Can you work these out from the model? Positions are in its coordinate system, mm. Face numbers are marked on the shaded views. A direction names the side the tool comes from. Round coordinates to 2 decimals unless told otherwise and drop trailing zeros. Loops run counter-clockwise (first coordinate to the right, second up) from the corner with the lowest first, then second, coordinate; pieces in that order, holes last. Notation, with made-up numbers: (-20, -37) -> (-3, -37) arc R12 cw to (-3, -28) -> close; hole circle Ø10 at (20, 22). An arc over 180 degrees is marked (long way). Write item = value, one per line.
Autodesk Inventor part; units mm, degrees
ref_plane "YZ Plane" through (0, 0, 0) normal (1, 0, 0) x (0, 1, 0)
ref_plane "XZ Plane" through (0, 0, 0) normal (0, 1, 0) x (-1, 0, 0)
ref_plane "XY Plane" through (0, 0, 0) normal (0, 0, 1) x (1, 0, 0)
sketch "Esquisse1" plane through (0, 0, 0) normal (0, 0, 1) x (1, 0, 0)
  line L0 (2, 0) -> (68, 0)
  line L1 (70, 2) -> (70, 28)
  line L2 (68, 30) -> (2, 30)
  line L3 (0, 28) -> (0, 2)
  arc A0 (2, 30) -> (0, 28) centre (2, 28) ccw
  arc A1 (70, 28) -> (68, 30) centre (68, 28) ccw
  arc A2 (68, 0) -> (70, 2) centre (68, 2) ccw
  arc A3 (0, 2) -> (2, 0) centre (2, 2) ccw
  point P0 (0, 0)
  point P1 (70, 30)
  point P2 (70, 0)
  point P3 (0, 30)
  dimension "d0" = 70
  dimension "d1" = 30
  dimension "d14" = 2
extrude "Extrusion1" add sketch "Esquisse1" along normal blind 5
sketch "Esquisse2" plane through (0, 0, 0) normal (-1, 0, 0) x (0, 0, 1)
  line L0 (5, 2) -> (5, 28)
  line L1 (5, 15) -> (5, 19)
  line L2 (5, 15) -> (5, 11)
  line L3 (5, 19) -> (11, 19)
  line L4 (13, 17) -> (13, 13)
  line L5 (11, 11) -> (5, 11)
  arc A0 (13, 17) -> (11, 19) centre (11, 17) ccw
  arc A1 (11, 11) -> (13, 13) centre (11, 13) ccw
  line L6 (5, 19) -> (12.4142, 11.5858) construction
  line L7 (5, 11) -> (12.4142, 18.4142) construction
  circle A2 centre (9, 15) radius 2.75
  line L8 (0, 2) -> (0, 28)
  line L9 (5, 2) -> (5, 28)
  line L10 (0, 2) -> (5, 2)
  line L11 (5, 28) -> (5, 2)
  line L12 (0, 28) -> (5, 28)
  line L13 (0, 2) -> (0, 28)
  line L14 (0, 2) -> (5, 2)
  line L15 (5, 28) -> (5, 2)
  line L16 (0, 28) -> (5, 28)
  line L17 (0, 2) -> (0, 28)
  line L18 (0, 28) -> (5, 28)
  line L19 (0, 2) -> (5, 2)
  point P0 (5, 0)
  point P1 (5, 30)
  point P2 (13, 19)
  dimension "d4" = 4
  dimension "d5" = 4
  dimension "d6" = 8
  dimension "d7" = 2
  dimension "d8" = 5.5
extrude "Extrusion2" add sketch "Esquisse2" against normal blind 5 contours L0 L3 A0 L4 A1 L5
sketch "Esquisse3" plane through (70, 0, 0) normal (1, 0, 0) x (0, 0, -1)
  line L0 (-11, 19) -> (-5, 19)
  line L1 (-5, 19) -> (-11, 19)
  line L2 (-11, 19) -> (-11, 19)
  line L3 (-13, 13) -> (-13, 17)
  line L4 (-13, 17) -> (-13, 13)
  line L5 (-11, 11) -> (-5, 11)
  line L6 (-5, 2) -> (-5, 28)
  line L7 (-5, 19) -> (-5, 11)
  arc A0 (-11, 19) -> (-13, 17) centre (-11, 17) ccw
  arc A1 (-13, 13) -> (-11, 11) centre (-11, 13) ccw
  circle A2 centre (-9, 15) radius 2.75
  circle A3 centre (-9, 15) radius 2.5
  point P0 (0, 0)
  point P1 (-13, 19)
  point P2 (-5, 0)
  point P3 (-5, 30)
  dimension "d11" = 2
extrude "Extrusion3" add sketch "Esquisse3" against normal blind 5 contours L0 L6 L5 A1 L3 A0
properties part number "Pied"
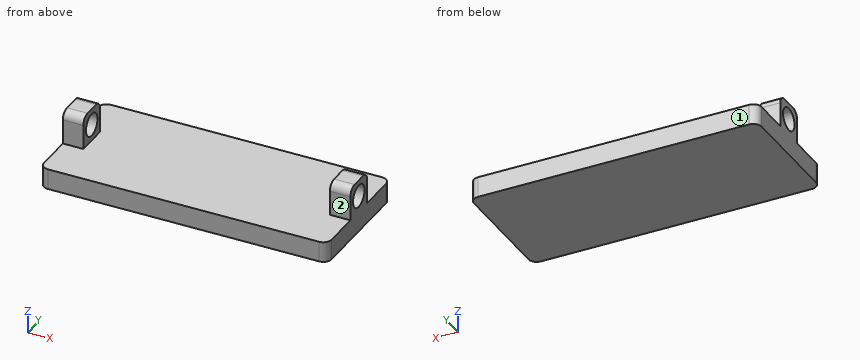
1. For the marked faces 1 and 2, which set-ups out of +Z, -Z, +X, -X, +Y, -Y let a thin tool reach every point of the face, with its end or its side?
Entries:
face_1 = +Z, -Z, +X, -X, +Y
face_2 = +Z, +X, -X, -Y
2. I need wall thicknesses on line 1 (X direction, y = 12.25, z = 11); line 2 (Y direction, x = 68.9, z = 9); line 3 (Z direction, x = 22, y = 15). Which ranges of each line are inside material? Lowest first, please. Write a range as [from, to].
Entries:
line_1 = [0, 5], [65, 70]
line_2 = [11, 12.25], [17.75, 19]
line_3 = [0, 5]
3. Suppose I cut it at A-A, the plane y = 15. List the corners of the cut face in (x, z) for me, and give its area (3 significant figures).
Entries:
outline = (0, 0) -> (70, 0) -> (70, 6.25) -> (65, 6.25) -> (65, 5) -> (5, 5) -> (5, 6.25) -> (0, 6.25) -> close; (0, 11.75) -> (5, 11.75) -> (5, 13) -> (0, 13) -> close; (65, 11.75) -> (70, 11.75) -> (70, 13) -> (65, 13) -> close
area = 375 mm²
4. Suppose I cut it at B-B, the plane z = 9. List the corners of the cut face in (x, y) for me.
Entries:
outline = (0, 11) -> (5, 11) -> (5, 12.25) -> (0, 12.25) -> close; (0, 17.75) -> (5, 17.75) -> (5, 19) -> (0, 19) -> close; (65, 11) -> (70, 11) -> (70, 12.25) -> (65, 12.25) -> close; (65, 17.75) -> (70, 17.75) -> (70, 19) -> (65, 19) -> close
5. Suppose I cut it at C-C, the plane x = 29.5. List the corners of the cut face in (y, z) for me.
Entries:
outline = (0, 0) -> (30, 0) -> (30, 5) -> (0, 5) -> close
6. Suppose I cut it at D-D, the plane y = 5.25. List the corners of the cut face in (x, z) for me, and give its area (3 significant figures).
Entries:
outline = (0, 0) -> (70, 0) -> (70, 5) -> (0, 5) -> close
area = 350 mm²
7. I'm going to push flat-ended pins straight in: pin 1 (4 mm diameter, centred on x = 3.5, z = 9.5, fed in from -Y); pin 2 (9 mm diameter, centred on x = 33.5, y = 17, fed in from +Z); pin 3 (2.5 mm diameter, centred on x = 67.5, z = 8.5, fed in from +Y); pin 4 (5.5 mm diameter, centred on x = 1.5, z = 7, fed in from +Y). Where does each tip first touch, or does it pass through?
Entries:
pin_1 = 11
pin_2 = 5
pin_3 = 19
pin_4 = 30
